Geometry: final body of the model. Coordinates: model frame, mm. Face numbers are marked on the shaded views. A direction names the side the tool comes from. Coordinates: 2 decimals unless noted, no trailing zeros. Loops run counter-clockwise (first coordinate to the right, second up) from the corner with the lowest first, then second, coordinate; pieces in that order, holes last. Notation, with made-up numbers: M 50.5,81 L 75.5,81 A18 ccw 75.5,94 Z; hole C 53.5,4.25 d8. An arc over 180 degrees is marked long. Write item = value, one per line. Start each with the question number.
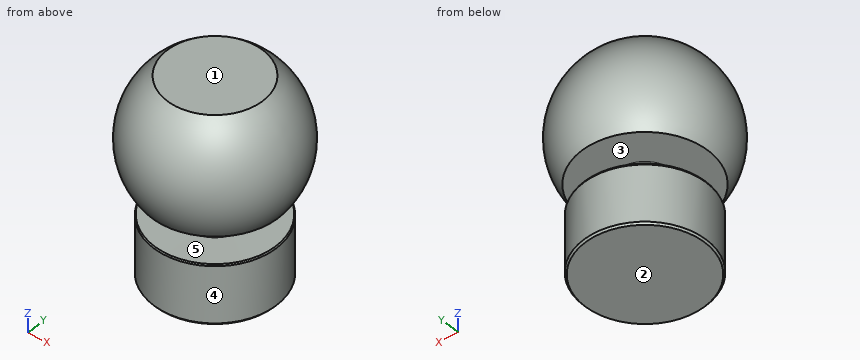
```python
from build123d import *


with BuildPart() as part:
    # Sketch1 → Revolve1 (revolve)
    with BuildSketch(Plane(origin=(0, 0, 0), x_dir=(1, 0, 0), z_dir=(0, 1, 0))):
        with BuildLine():
            Line((18.554185143, -2.529876216), (28.121974873, -2.529876216))
            Line((28.121974873, -2.529876216), (33.621974873, -2.529876216))
            Line((33.621974873, -2.529876216), (34.121974873, -3.147134349))
            Line((34.121974873, -3.147134349), (34.121974873, -16.947673594))
            Line((34.121974873, -16.947673594), (34.121974873, -21.529876216))
            Line((34.121974873, -21.529876216), (33.871974873, -22.029876216))
            Line((33.871974873, -22.029876216), (23.525737468, -21.994577645))
            ThreePointArc((23.525737468, -21.994577645), (21.818442704, -22.783035248), (21.121974873, -24.529876216))
            Line((21.121974873, -24.529876216), (21.121974873, -29.529876216))
            ThreePointArc((21.121974873, -29.529876216), (21.70776131, -30.944089778), (23.121974873, -31.529876216))
            Line((23.121974873, -31.529876216), (23.163890071, -31.529876216))
            Line((23.163890071, -31.529876216), (25.892484704, -31.529876216))
            Line((25.892484704, -31.529876216), (34.707125886, -31.529876216))
            ThreePointArc((34.707125886, -31.529876216), (39.275357094, -50.049169414), (29.672271119, -66.529876216))
            Line((29.672271119, -66.529876216), (19.091113774, -66.529876216))
            Line((19.091113774, -66.529876216), (14.121974873, -66.529876216))
            Line((14.121974873, -66.529876216), (14.121974873, -2.529876216))
            Line((14.121974873, -2.529876216), (18.554185143, -2.529876216))
        make_face()
    revolve(axis=Axis((14.121974873, 0, 2.529876216), (0, 0, 1)))


solid = part.part
```
Item 1: Section query B-B (z = 25.5). Return the cut outline in (x, y).
Item 2: First-contact query: pin 1 (5 mm diameter, centred on y = -19.5, z = 39, fed in from -X); pin 2 (1.5 mm diameter, centred on x = 8, y = -17.5, fed in from +Z); pin 3 (8 mm diameter, centred on x = -3, z = 13, fed in from +Y); pin 4 (10 mm diameter, centred on x = -2, y = -11, fed in from +Z). Flat tips, straight axial feed; report the tip coordinate or a pass-through.
Item 3: Pull-direction query (Z, two-part tool) for the marked faces 1, 2 and 3; classes: released by +Z, released by -Z, zero draft, split by the parting line, or undercut.
Item 4: Section query C-C (z = 56.5). Return the cut outline in (x, y), plus the area to 3 significant figures.
Item 5: Line query: line 1 (Z direction, x = 2, y = 2.5); line 2 (Z direction, x = -3.5, y = 6.5); line 3 (X direction, y = -16, z = 46.5). Output: solid intervals per line, ascending. Write a range as from..to.
Item 6: Reachability of the marked faces 4 and 5 from +Z, -Z, +X, -X, +Y, -Y: full face, straight path, thin tool, end or side. Return the list, or none.
Item 7: Section query A-A (y = 0). Return the cut outline in (x, z).
Verdict:
q1.outline = C 14.12,0 d14
q2.pin_1 = -3.44
q2.pin_2 = 64.58
q2.pin_3 = 15.09
q2.pin_4 = 66.53
q3.face_1 = released by +Z
q3.face_2 = released by -Z
q3.face_3 = undercut
q4.outline = C 14.12,0 d46.66
q4.area = 1,710 mm2
q5.line_1 = 2.53..22, 31.53..66.53
q5.line_2 = 2.53..22.03, 31.53..63.55
q5.line_3 = -5.62..33.86
q6.face_4 = -Z
q6.face_5 = none
q7.outline = M -6.46,31.53 L 5.12,31.53 A2 cw 7.12,29.53 L 7.12,24.53 A2.54 cw 4.72,21.99 L -5.63,22.03 L -5.88,21.53 L -5.88,3.15 L -5.38,2.53 L 33.62,2.53 L 34.12,3.15 L 34.12,21.53 L 33.87,22.03 L 23.53,21.99 A2.54 cw 21.12,24.53 L 21.12,29.53 A2 cw 23.12,31.53 L 34.71,31.53 A25.41 ccw 29.67,66.53 L -1.43,66.53 A25.41 ccw Z
